Job drawing, mm, ordinate dimensions from the low corner. One solid piece. A direction names the side the tool comes from. Round coordinates to 2 decimals unless told otherwise and drop trailing zeros. Loops run counter-clockwise (first coordinate to the right, second up) from the corner with the lowest first, then second, coordinate; pieces in that order, holes last.
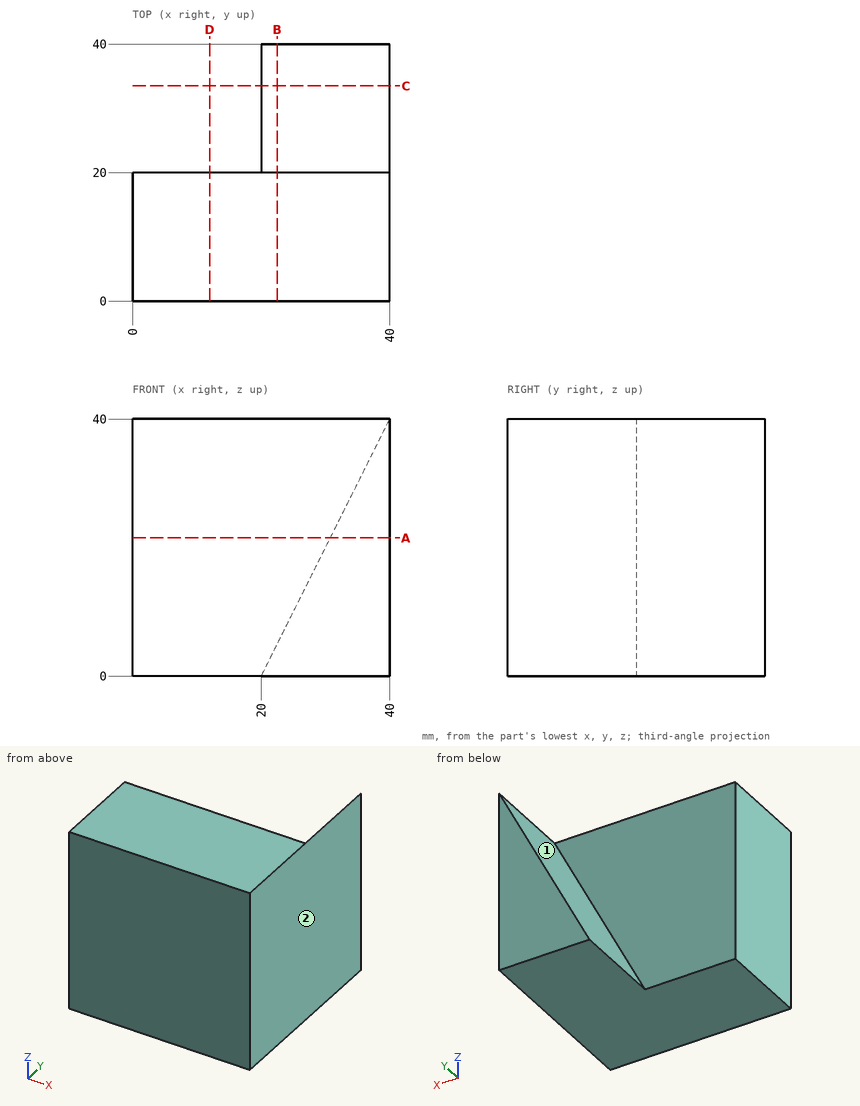
1) Tool access for the marked faces 1 and 2: list every direction of +Z, -Z, +X, -X, +Y, -Y with a clear straight run to the whole face (end or side of a thin tool).
Values:
face 1: +Z, -X, +Y
face 2: +Z, -Z, +X, +Y, -Y
2) Slice it at A-A, the plane z = 21.5. Give the cut face in (x, y).
Values:
outline: (0, 0) - (40, 0) - (40, 40) - (30.75, 40) - (30.75, 20) - (0, 20) - close
3) Slice it at B-B, the plane x = 22.5. Give the cut face in (y, z).
Values:
outline: (0, 0) - (40, 0) - (40, 5) - (20, 5) - (20, 40) - (0, 40) - close
4) Drop flat-ended pins along their axis: pin 1 Ø12 at (x, y) = (5.5, 27.5) entering from -Z; pin 2 Ø4 at (x, z) = (22, 24.5) entering from +Y; pin 3 Ø1.5 at (y, z) = (22, 33.5) entering from -X (3 decimals); pin 4 Ø4 at (x, y) = (20.5, 32.5) entering from +Z. Give the stop position or say it passes through.
Values:
pin 1: passes through
pin 2: stops at y = 20
pin 3: stops at x = 36.375
pin 4: stops at z = 5
5) Slice it at C-C, the plane y = 33.5. Give the cut face in (x, z).
Values:
outline: (20, 0) - (40, 0) - (40, 40) - close
6) Wall check: line 1 along Y through (x, z) = (10, 6); line 2 along X through (y, z) = (38, 24); line 3 along X through (y, z) = (35, 30). Give the ranges that are in metal, low to high.
Values:
line 1: y = 0 to 20
line 2: x = 32 to 40
line 3: x = 35 to 40
7) Slice it at D-D, the plane x = 12. Give the cut face in (y, z).
Values:
outline: (0, 0) - (20, 0) - (20, 40) - (0, 40) - close
